Answer from the drawing. Dimensions are ordinates in mm from the lowest x, y and z of the part. A direction names the side the tool comes from. Coordinates: 2 decimals unless noted, no trailing zeros. Write each loop counter-clockwise with the first axis right and the second up, starting at its lowest first coordinate (ties: lowest second). Pieces come first, ordered by that corner, then holes. Notation, with made-up numbers: (-25.5, -8) -> (29.5, -8) arc R17 cw to (29.5, 8) -> close; hole circle Ø8 at (-9.5, 75.5). An arc over 180 degrees is marked (long way). One line per item, written item: value. Start each with the question number.
1. For the marked faces 1, 2, 3, 4 and 5, determine the directions among +Z, -Z, +X, -X, +Y, -Y from which every point of the face is accessible in a straight line to the end or side of a thin tool.
2. Find section A-A, the plane x = 127. Write down the section's boundary in (y, z), and give its area (3 significant figures).
3. For a pull along Z with two mould halves and no side action, classify the marked faces 6, 7 and 8 as pulls with the +Z half, pulls with the -Z half, needs draft (parallel to the pull), parting line crosses it, or undercut.
4. Given P1, Ø4, axis at x = 56, z = 140, coming from the -Y side; P2, Ø12, axis at y = 29, z = 182.5, coming from the -X side (1 decimal); P3, Ø3, axis at y = 98.5, z = 172, coming from the +X side, each flat-ended and moving along its own axis, determine where each tip first touches the part or whether it passes through.
5. Find section D-D, the plane x = 29. Write down the section's boundary in (y, z).
6. Consider line 1 along Z through (x, y) = (156, 100.5); line 2 along Z through (x, y) = (101, 85.5); line 3 along Z through (x, y) = (127, 65). Determine where each line is inside the solid, lowest interval first.
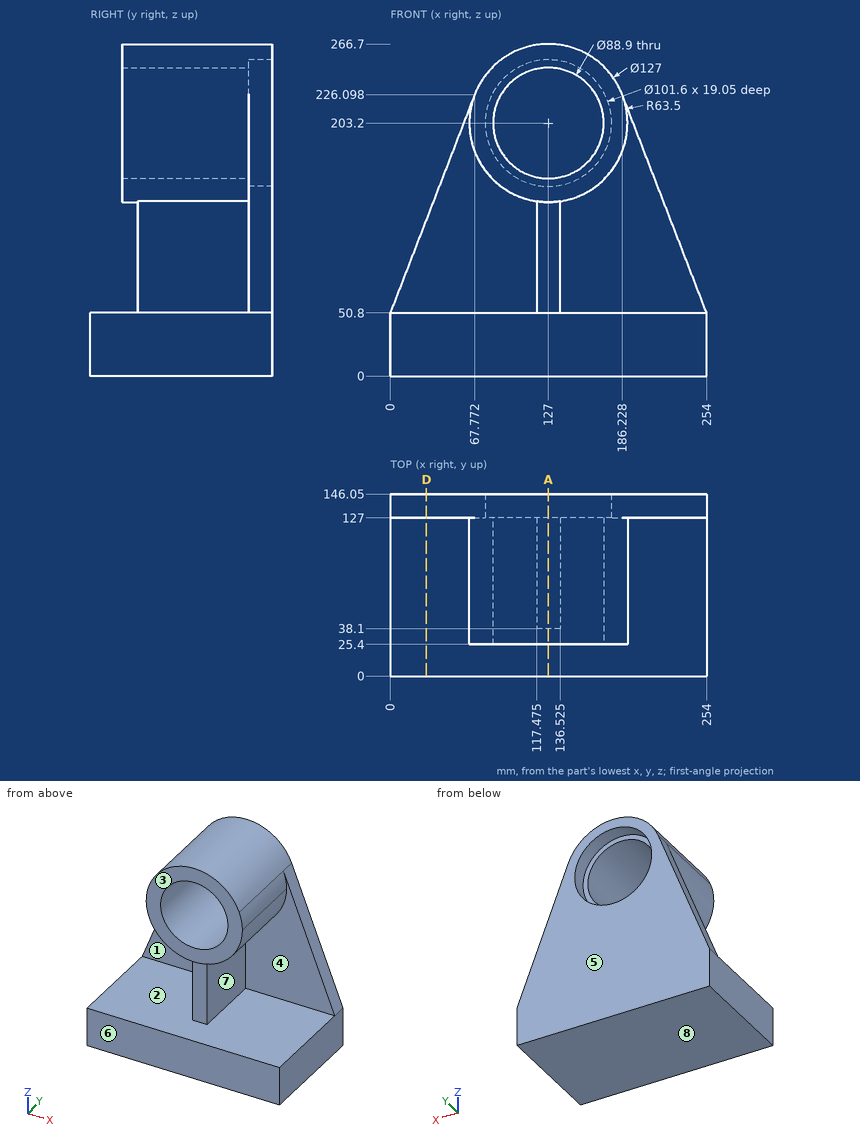
Answer block:
1. face 1: -X, -Y
1. face 2: -Y
1. face 3: +Z, +X, -X, -Y
1. face 4: +X, -Y
1. face 5: +Z, -Z, +X, -X, +Y
2. outline: (0, 0) -> (146.05, 0) -> (146.05, 152.4) -> (127, 152.4) -> (127, 158.75) -> (25.4, 158.75) -> (25.4, 139.7) -> (38.1, 139.7) -> (38.1, 50.8) -> (0, 50.8) -> close; (25.4, 247.65) -> (127, 247.65) -> (127, 254) -> (146.05, 254) -> (146.05, 266.7) -> (25.4, 266.7) -> close
2. area: 21,400 mm2
3. face 6: needs draft
3. face 7: undercut
3. face 8: pulls with the -Z half
4. P1: stops at y = 127
4. P2: stops at x = 65.2
4. P3: stops at x = 183.13
5. outline: (0, 0) -> (146.05, 0) -> (146.05, 125.81) -> (127, 125.81) -> (127, 50.8) -> (0, 50.8) -> close
6. line 1: z = 0 to 50.8, 146.71 to 169.51, 236.89 to 259.69
6. line 2: z = 0 to 50.8, 145.27 to 167.15, 239.25 to 261.13
6. line 3: z = 0 to 158.75, 247.65 to 266.7
